Part print with two shaded views. Sizes in mm from the minimum x, y, z corner. Coordinates: 2 decimals unless noted, no trailing zeros. Write each loop counter-clockwise with the first axis right and the second up, starting at its lowest first coordinate (ties: lowest second). Pieces come first, ordered by that corner, then holes.
Q1. Band-saw the part on C-C, the plane y = 1.75. Write the cut outline in (x, z).
Q2. Pin check, flat tip, straight feed: P1, Ø6.5, axis at y = 9, z = 9, coming from the -X side. Stop position of the tip, or through.
Q3. Band-saw the part on B-B, the plane z = 8.5. Write the cut outline in (x, y).
Q4. Pull direction Y, two halves, no side cores. Call the marked faces 1, 2, 3 and 4: released by +Y, released by -Y, zero draft, split by the parting line, or undercut.
Q5. Drill centre lines: probe 1 along Z at (x, y) = (4.15, 11.25); probe 2 along Y at (x, z) = (3.6, 40); probe 3 along Y at (x, z) = (2.6, 9). Where is each one in solid material? Low to high.
Q6. Band-saw the part on A-A, the plane y = 9. Write the cut outline in (x, z).
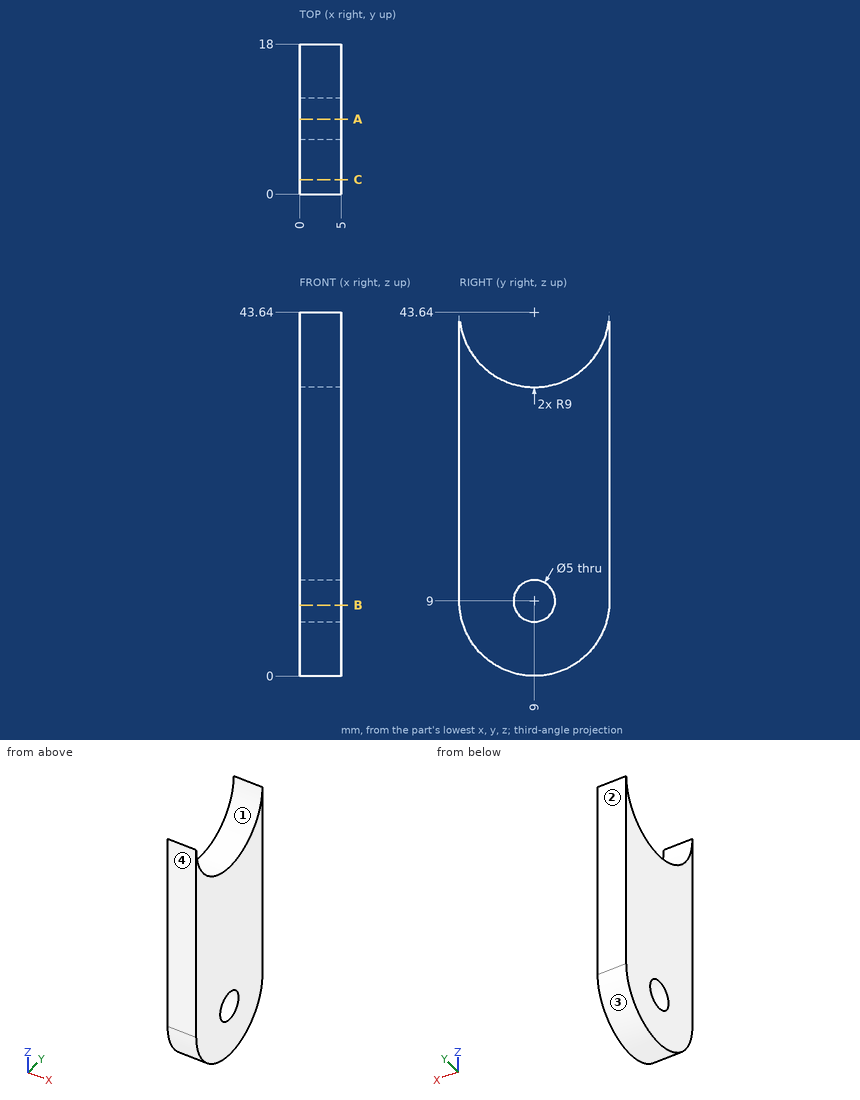
Answer sheet:
1. outline: (0, 3.67) - (5, 3.67) - (5, 38.31) - (0, 38.31) - close
2. P1: stops at x = 0
3. outline: (0, 0.01) - (5, 0.01) - (5, 6.55) - (0, 6.55) - close; (0, 11.45) - (5, 11.45) - (5, 17.99) - (0, 17.99) - close
4. face 1: undercut
4. face 2: released by +Y
4. face 3: split by the parting line
4. face 4: released by -Y
5. probe 1: z = 0.29 to 7.91, 10.09 to 34.93
5. probe 2: y = 0 to 0.77, 17.23 to 18
5. probe 3: y = 0 to 6.5, 11.5 to 18
6. outline: (0, 0) - (5, 0) - (5, 6.5) - (0, 6.5) - close; (0, 11.5) - (5, 11.5) - (5, 34.64) - (0, 34.64) - close
